Read the model definition and answer for the solid it produces. Units are mm, in the model's axes. A direction names the side the tool comes from. Coordinates: 2 decimals unless noted, no trailing zeros. Loops run counter-clockwise (first coordinate to the right, second up) from the corner with the lowest first, then second, coordinate; pieces in that order, holes last.
Q1. Straight lines are drawn through the part: line 1 (Y direction, x = -26, z = 42.5); line 2 (X direction, y = 18.5, z = 16.5) (3 decimals); line 3 (Z direction, x = -22, y = -13). For each, find the intervals that lie inside material, in ascending order.
Q2. The mould has two halves that part along X. Classify faces 4 (the face through (-1, -50.8, 32)), 5 (the face through (-1, -63.5, 25)), 6 (the face through (84.455, -1, 25)): pulls with the +X half, pulls with the -X half, needs draft (parallel to the pull), parting line crosses it, or undercut.
Q3. Section A-A (y = 38) is taken. Give the vertices of the cut face in (x, z) (3 decimals), then the cut area to 3 significant figures.
Q4. Section D-D (z = 27) is taken. Give the vertices of the cut face in (x, y) (3 decimals), then the cut area to 3 significant figures.
Q5. Section C-C (x = 64) is taken. Give the vertices of the cut face in (y, z).
Q6. Flat-ended cylindrical pins translate along their axes: P1, Ø3, axis at x = 5.5, y = -29, coming from the -Z side; P2, Ø1, axis at x = 15, y = -33, coming from the +Z side; P3, Ø16.5, axis at x = 20.72, z = 23.86, coming from the -Y side. Find the tip coordinate at first contact, or state that the pin passes through.
Q7. Which of the six approach directions +Z, -Z, +X, -X, +Y, -Y give full straight-line access (tool end or side, diameter ignored) to faces 1 (the face through (71.755, -1, 32)), 2 (the face through (14.026, -57.239, 29.999)), 3 (the face through (-1, 63.5, 25))?
Q8. Section B-B (z = 41) is taken. Give the vertices of the cut face in (x, y) (3 decimals).
from build123d import *

# Parameters (mm, degrees)
F0_W     = 168.91
F0_H     = 127
F1_DEPTH = 50.8
F2_W     = 143.51
F2_H     = 101.6
F3_DEPTH = 38.1
F4_R     = 9.076536
F5_DEPTH = 25.4


with BuildPart() as f1:
    # F0 (on Top) → F1 (new body)
    with BuildSketch(Plane.XY):
        Rectangle(F0_W, F0_H)
    extrude(amount=F1_DEPTH)

    # F2 (on face) → F3 (cut)
    with BuildSketch(Plane.XY.offset(50.8)):
        Rectangle(F2_W, F2_H)
    extrude(amount=-F3_DEPTH, mode=Mode.SUBTRACT)

    # F4 (on face) → F5 (cut)
    with BuildSketch(Plane.XZ.offset(63.5)):
        with Locations((20.715535, 23.864772)):
            Circle(F4_R)
    extrude(amount=-F5_DEPTH, mode=Mode.SUBTRACT)


solid = f1.part
Numbers:
1. line 1: y = -63.5 to -50.8, 50.8 to 63.5
1. line 2: x = -84.455 to -71.755, 71.755 to 84.455
1. line 3: z = 0 to 12.7
2. face 4: undercut
2. face 5: needs draft
2. face 6: pulls with the +X half
3. outline: (-84.455, 0) - (84.455, 0) - (84.455, 50.8) - (71.755, 50.8) - (71.755, 12.7) - (-71.755, 12.7) - (-71.755, 50.8) - (-84.455, 50.8) - close
3. area: 3,110 mm2
4. outline: (-84.455, -63.5) - (12.198, -63.5) - (12.198, -50.8) - (-71.755, -50.8) - (-71.755, 50.8) - (71.755, 50.8) - (71.755, -50.8) - (29.233, -50.8) - (29.233, -63.5) - (84.455, -63.5) - (84.455, 63.5) - (-84.455, 63.5) - close
4. area: 6,650 mm2
5. outline: (-63.5, 0) - (63.5, 0) - (63.5, 50.8) - (50.8, 50.8) - (50.8, 12.7) - (-50.8, 12.7) - (-50.8, 50.8) - (-63.5, 50.8) - close
6. P1: stops at z = 0
6. P2: stops at z = 12.7
6. P3: stops at y = 50.8
7. face 1: +Z
7. face 2: -Y
7. face 3: +Z, -Z, +X, -X, +Y
8. outline: (-84.455, -63.5) - (84.455, -63.5) - (84.455, 63.5) - (-84.455, 63.5) - close; hole (-71.755, -50.8) - (71.755, -50.8) - (71.755, 50.8) - (-71.755, 50.8) - close
